```python
from build123d import *

# Parameters (mm, degrees)
SKETCH1_W           = 50.8
SKETCH1_H           = 20.32
SKETCH1_R           = 1.4732
BOSS_EXTRUDE1_DEPTH = 4.826
SKETCH2_W           = 50.8
SKETCH2_H           = 4.826
BOSS_EXTRUDE2_DEPTH = 26.924
FILLET1_R           = 2.54
SKETCH3_R           = 1.4732
SKETCH3_R_2         = 4.8133
CUT_EXTRUDE1_DEPTH  = 26.924


with BuildPart() as part:
    # Sketch1 → Boss-Extrude1 (new body)
    with BuildSketch(Plane(origin=(0, 0, 0), x_dir=(1, 0, 0), z_dir=(0, 1, 0))):
        with Locations((25.4, 10.16)):
            Rectangle(SKETCH1_W, SKETCH1_H)
        with Locations(Location((12.7, 10.16, 0), (0, 0, 270))):
            Circle(SKETCH1_R, mode=Mode.SUBTRACT)
        with Locations(Location((38.1, 10.16, 0), (0, 0, 270))):
            Circle(SKETCH1_R, mode=Mode.SUBTRACT)
    extrude(amount=BOSS_EXTRUDE1_DEPTH)

    # Sketch2 → Boss-Extrude2 (add)
    with BuildSketch(Plane(origin=(0, 4.826, 0), x_dir=(1, 0, 0), z_dir=(0, 1, 0))):
        with Locations((25.4, 17.907)):
            Rectangle(SKETCH2_W, SKETCH2_H)
    extrude(amount=BOSS_EXTRUDE2_DEPTH)

    # Fillet1
    fillet1_edges = [part.edges().sort_by_distance(p)[0] for p in [
        (25.4, 31.75, -15.494),
        (25.4, 4.826, 0),
    ]]
    fillet(fillet1_edges, radius=FILLET1_R)

    # Sketch3 → Cut-Extrude1 (cut)
    with BuildSketch(Plane(origin=(0, 0, -20.32), x_dir=(-1, 0, 0), z_dir=(0, 0, -1))):
        with Locations((-38.1, 19.05)):
            Circle(SKETCH3_R)
        with Locations((-12.7, 19.05)):
            Circle(SKETCH3_R)
        with Locations((-25.4, 19.05)):
            Circle(SKETCH3_R_2)
    extrude(amount=-CUT_EXTRUDE1_DEPTH, mode=Mode.SUBTRACT)


solid = part.part
```
Source: CAD feature listing. Evaluate the final solid. Frame: model axes, mm. A direction names the side the tool comes from. Round coordinates to 2 decimals unless told otherwise and drop trailing zeros. Loops run counter-clockwise (first coordinate to the right, second up) from the corner with the lowest first, then second, coordinate; pieces in that order, holes last.
1. Section query A-A on y = 19.05. Output: boundary loops of the cut face in (x, z), and give its area (3 significant figures).
2. Section query B-B on x = 25.4. Output: boundary loops of the cut face in (y, z).
3. Access query for faces 1 (the flat face through (25, 4.826, -9)), 2 (the flat face through (0, 12, -16)). Directions: +Z, -Z, +X, -X, +Y, -Y. A direction counts if a zero-diameter tool reaches every point of the face in a straight line with its end or side. Return the directions, or none.
4. Section query D-D on x = 12.7. Output: boundary loops of the cut face in (y, z), and give its area (3 significant figures).
5. Mould query, pull axis Y, two halves, no side actions, for faces 3 (the cylindrical face through (25.76, 31.03, -16.26)), 4 (the cylindrical face through (39.186, 20.046, -17.941)), 5 (the flat face through (25, 14, -15.494)), 6 (the cylindrical face through (11.295, 19.493, -17.941)). Classes: released by +Y, released by -Y, zero draft, split by the parting line, or undercut.
6. Contact query for flat-ended pins moving along their axis: pin 1 (10.5 mm diameter, centred on x = 32, z = -7, fed in from +Y); pin 2 (2.5 mm diameter, centred on x = 38.1, y = 19.05, fed in from +Z); pin 3 (15.5 mm diameter, centred on x = 25.4, y = 19.05, fed in from +Z). Output: stop coordinate, or through.
7. Ray query, L1, parallel to X at y = 1.8, z = -10.16; L2, parallel to Y at x = 22, z = -13.25; L3, parallel to Y at x = 12.7, z = -17.55. Return the intervals inside material, ascending.
8. Section query C-C on z = -17. Output: boundary loops of the cut face in (x, y), and give its area (3 significant figures).
Answers below:
1. outline: (0, -20.32) - (11.23, -20.32) - (11.23, -15.49) - (0, -15.49) - close; (14.17, -20.32) - (20.59, -20.32) - (20.59, -15.49) - (14.17, -15.49) - close; (30.21, -20.32) - (36.63, -20.32) - (36.63, -15.49) - (30.21, -15.49) - close; (39.57, -20.32) - (50.8, -20.32) - (50.8, -15.49) - (39.57, -15.49) - close
1. area: 170 mm2
2. outline: (0, -20.32) - (14.24, -20.32) - (14.24, -15.49) - (4.83, -15.49) - (4.83, -2.54) arc R2.54 ccw to (2.29, 0) - (0, 0) - close; (23.86, -20.32) - (31.75, -20.32) - (31.75, -18.03) arc R2.54 ccw to (29.21, -15.49) - (23.86, -15.49) - close
3. face 1: +Z, +X, -X, +Y
3. face 2: +Z, -Z, -X, +Y, -Y
4. outline: (0, -20.32) - (17.58, -20.32) - (17.58, -15.49) - (4.83, -15.49) - (4.83, -11.63) - (0, -11.63) - close; (0, -8.69) - (4.83, -8.69) - (4.83, -2.54) arc R2.54 ccw to (2.29, 0) - (0, 0) - close; (20.52, -20.32) - (31.75, -20.32) - (31.75, -18.03) arc R2.54 ccw to (29.21, -15.49) - (20.52, -15.49) - close
4. area: 197 mm2
5. face 3: released by +Y
5. face 4: undercut
5. face 5: zero draft
5. face 6: undercut
6. pin 1: stops at y = 4.83
6. pin 2: passes through
6. pin 3: stops at z = -15.49
7. L1: x = 0 to 11.23, 14.17 to 36.63, 39.57 to 50.8
7. L2: y = 0 to 4.83
7. L3: y = 0 to 17.58, 20.52 to 31.7
8. outline: (0, 0) - (50.8, 0) - (50.8, 31.53) - (0, 31.53) - close; hole circle Ø2.95 at (12.7, 19.05); hole circle Ø9.63 at (25.4, 19.05); hole circle Ø2.95 at (38.1, 19.05)
8. area: 1,520 mm2
